Here's how the part is built. I have some questions about the finished solid (model axes, mm). A direction names the side the tool comes from. Coordinates: 2 decimals unless noted, no trailing zeros. Write each loop counter-clockwise with the first axis right and the second up, starting at its lowest first coordinate (ties: lowest second). Pieces come first, ordered by that corner, then holes. Notation, with made-up numbers: (69, 34.25) -> (116, 34.25) arc R23 cw to (116, 47.25) -> close; hole circle Ø7 at (11, -10). An arc over 180 degrees is marked (long way). Use a Markdown table: item, result. Add a question column.
Item 1: Will these pins go through, and if not, where does the flat tip stop? pin 1 Ø4 at (x, z) = (80.5, -6.5) entering from +Y; pin 2 Ø1.3 at (x, y) = (141.5, 9) entering from -Z; pin 3 Ø5 at (x, y) = (19, 14) entering from +Z.
Item 2: If I drill on line 1 along X through (y, z) = (0.35, 0); line 2 along Z through (x, y) = (35, 10.5); line 3 along Z through (x, y) = (78.5, 7.5), over which ranges is the centre line in solid material (lowest first)? Write a range as from..to.
Item 3: Imagine slicing it at B-B, the plane y = 16.5. Write out the boundary of the cut face in (x, z) (1 decimal).
Item 4: Imagine slicing it at A-A, the plane x = 106. Write out the boundary of the cut face in (y, z) (1 decimal), and give its area (3 significant figures).
Item 5: On a 3-axis mill with a long thin cutter (end or side, diameter ignored), from which of +Z, -Z, +X, -X, +Y, -Y can I reach the whole of each face in a straight line? I mean faces 5 (the flat face through (70, 10, -6.528)), 6 (the cylindrical face through (-10.38, 5.66, 7.59)), 7 (the cylindrical face through (133.184, 12.93, 7.146)). Say none if no direction works.
Item 6: If we mould it in two halves opening along Y, with no side actions, what happens to faces 1 (the flat face through (138, 18.136, 7)), 2 (the flat face through (140.64, 9, -3)), 3 (the flat face through (39, 7, -6.972)), 4 (the flat face through (38, 7, 6.972))? For each: pulls with the +Y half, pulls with the -Y half, needs draft (parallel to the pull), parting line crosses it, or undercut.
```python
from build123d import *

# Parameters (mm, degrees)
BOSS_EXTRUDE1_DEPTH          = 7.747
BOSS_EXTRUDE2_DEPTH          = 8.1915
SHELL1_START                 = 1.2192
SHELL1_DEPTH                 = 16.9164
CUT_EXTRUDE1_DEPTH           = 1.2192
EXTRUDE_THIN1_START          = -16.383
SKETCH4_W                    = 128.27
SKETCH4_H                    = 1.27
EXTRUDE_THIN1_DEPTH          = 16.383
FILLET1_R                    = 2.54
SKETCH5_W                    = 13.9446
SKETCH5_H                    = 1.27
CUT_EXTRUDE2_DEPTH           = 129.4892
F_3_4_0_162_DIAMETER_HOLE1_D = 4.1148
CUT_EXTRUDE3_REACH           = 145.248
FILLET2_DEPTH                = 18.1356
CUT_EXTRUDE4_REACH           = 145.099
SKETCH9_R                    = 2.9591
FILLET3_R                    = 0.635
FILLET4_R                    = 2.54


with BuildPart() as part:
    # Sketch1 → Boss-Extrude1 (new, symmetric)
    with BuildSketch(Plane.XY):
        with BuildLine():
            Line((0, 0), (141.859, 0))
            Line((141.859, 0), (141.859, 18.1356))
            Line((141.859, 18.1356), (133.9088, 18.1356))
            Line((133.9088, 18.1356), (133.9088, 12.1666))
            Line((133.9088, 12.1666), (129.615181762, 12.1666))
            ThreePointArc((129.615181762, 12.1666), (128.080397702, 13.170161892), (128.3843, 14.978570578))
            ThreePointArc((128.3843, 14.978570578), (128.72346749, 16.699838275), (127.341060995, 17.78))
            Line((127.341060995, 17.78), (124.186037439, 18.1356))
            Line((124.186037439, 18.1356), (121.646037439, 18.1356))
            Line((121.646037439, 18.1356), (108.629212725, 15.24))
            Line((108.629212725, 15.24), (8.934212725, 15.24))
            Line((8.934212725, 15.24), (0, 12.7))
            Line((0, 12.7), (0, 0))
        make_face()
    extrude(amount=BOSS_EXTRUDE1_DEPTH, both=True)

    # Sketch2 → Boss-Extrude2 (add, symmetric)
    with BuildSketch(Plane.XY):
        with BuildLine():
            Line((0, 12.7), (-7.024172619, 10.703025112))
            ThreePointArc((-7.024172619, 10.703025112), (-10.369324418, 5.571014033), (-5.748264059, 1.5494))
            Line((-5.748264059, 1.5494), (0, 1.5494))
            Line((0, 1.5494), (0, 12.7))
        make_face()
    extrude(amount=BOSS_EXTRUDE2_DEPTH, both=True)

    # Shell1: read off the stored shape, not the designer's step
    # Shell1 outline → Shell1 (cut)
    with BuildSketch(Plane(origin=(0, 0, 0), x_dir=(1, 0, 0), z_dir=(0, 1, 0)).offset(SHELL1_START)):
        Polygon((140.6398, -6.5278), (140.6398, 6.5278), (-1.2192, 6.5278), (-1.2192, 6.9723), (-12, 6.9723), (-12, -6.9723), (-1.2192, -6.9723), (-1.2192, -6.5278), align=None)
    extrude(amount=SHELL1_DEPTH, mode=Mode.SUBTRACT)

    # Sketch3 → Cut-Extrude1 (cut)
    with BuildSketch(Plane(origin=(141.859, 0, 0), x_dir=(0, 0, -1), z_dir=(1, 0, 0))):
        Polygon((-2.2225, 13.0556), (-0.635, 13.0556), (-0.635, 0), (0.635, 0), (0.635, 13.0556), (2.2225, 13.0556), (2.2225, 18.1356), (-2.2225, 18.1356), align=None)
    extrude(amount=-CUT_EXTRUDE1_DEPTH, mode=Mode.SUBTRACT)

    # Sketch4 → Extrude-Thin1 (add)
    with BuildSketch(Plane.XY.offset(8.1915).offset(EXTRUDE_THIN1_START)):
        with Locations((64.135, 7.1628)):
            Rectangle(SKETCH4_W, SKETCH4_H)
    extrude_thin1 = extrude(amount=EXTRUDE_THIN1_DEPTH)

    # Fillet1
    fillet1_edges = [part.edges().sort_by_distance(p)[0] for p in [
        (141.859, 9.0678, 7.747),
        (141.859, 9.0678, -7.747),
    ]]
    fillet(fillet1_edges, radius=FILLET1_R)

    # Mirror2: Extrude-Thin1 across plane
    add(extrude_thin1.mirror(Plane.XY))

    # Sketch5 → Cut-Extrude2 (cut)
    with BuildSketch(Plane.ZY.offset(1.2192)):
        with Locations((0, 7.1628)):
            Rectangle(SKETCH5_W, SKETCH5_H)
    extrude(amount=-CUT_EXTRUDE2_DEPTH, mode=Mode.SUBTRACT)

    # 3/4 (0.162) Diameter Hole1 (through all)
    with Locations(Plane(origin=(0, 0, -8.1915), x_dir=(-1, 0, 0), z_dir=(0, 0, -1))):
        with Locations((5.748264059, 6.215135941)):
            Hole(F_3_4_0_162_DIAMETER_HOLE1_D / 2)

    # Sketch8 → Cut-Extrude3 (cut, up to next)
    with BuildSketch(Plane.XZ, mode=Mode.PRIVATE) as cut_extrude3_sk1:
        Polygon((140.6398, -6.5278), (140.6398, 6.5278), (140.0048, 6.5278), (140.0048, 4.064), (133.9088, 4.064), (133.9088, -4.064), (140.0048, -4.064), (140.0048, -6.5278), align=None)
    cut_extrude3_tool1 = extrude(cut_extrude3_sk1.sketch, amount=-CUT_EXTRUDE3_REACH, mode=Mode.PRIVATE) & part.part
    add(cut_extrude3_tool1.solids().sort_by_distance((137.439195, 0, 0))[0], mode=Mode.SUBTRACT)

    # Fillet2: read off the stored shape, not the designer's step
    # Fillet2 outline → Fillet2 (add)
    with BuildSketch(Plane(origin=(0, 0, 0), x_dir=(1, 0, 0), z_dir=(0, 1, 0))):
        with BuildLine():
            ThreePointArc((140.0048, 6.5278), (140.453812806, 6.341812806), (140.6398, 5.8928))
            Line((140.6398, 5.8928), (140.6398, 6.5278))
            Line((140.6398, 6.5278), (140.0048, 6.5278))
        make_face()
        with BuildLine():
            Line((140.6398, -6.5278), (140.6398, -5.8928))
            ThreePointArc((140.6398, -5.8928), (140.453812806, -6.341812806), (140.0048, -6.5278))
            Line((140.0048, -6.5278), (140.6398, -6.5278))
        make_face()
    extrude(amount=FILLET2_DEPTH)

    # Sketch9 → Cut-Extrude4 (cut, up to next)
    with BuildSketch(Plane(origin=(0, 1.2192, 0), x_dir=(1, 0, 0), z_dir=(0, 1, 0)), mode=Mode.PRIVATE) as cut_extrude4_sk1:
        with Locations(Location((119.9388, 0, 0), (0, 0, 270))):
            Circle(SKETCH9_R)
    cut_extrude4_tool1 = extrude(cut_extrude4_sk1.sketch, amount=-CUT_EXTRUDE4_REACH, mode=Mode.PRIVATE) & part.part
    # Sketch9 → Cut-Extrude4 (cut, up to next)
    with BuildSketch(Plane(origin=(0, 1.2192, 0), x_dir=(1, 0, 0), z_dir=(0, 1, 0)), mode=Mode.PRIVATE) as cut_extrude4_sk2:
        with Locations(Location((6.985, 0, 0), (0, 0, 270))):
            Circle(SKETCH9_R)
    cut_extrude4_tool2 = extrude(cut_extrude4_sk2.sketch, amount=-CUT_EXTRUDE4_REACH, mode=Mode.PRIVATE) & part.part
    add(cut_extrude4_tool1.solids().sort_by_distance((119.9388, 1.2192, 0))[0], mode=Mode.SUBTRACT)
    add(cut_extrude4_tool2.solids().sort_by_distance((6.985, 1.2192, 0))[0], mode=Mode.SUBTRACT)

    # Fillet3
    fillet3_edges = [part.edges().sort_by_distance(p)[0] for p in [
        (141.859, 0, -2.921),
        (69.6595, 0, -7.747),
        (141.859, 0, 2.921),
        (141.115051224, 0, 7.003051224),
        (141.115051224, 0, -7.003051224),
        (69.6595, 0, 7.747),
    ]]
    fillet(fillet3_edges, radius=FILLET3_R)

    # Fillet4
    fillet4_edges = [part.edges().sort_by_distance(p)[0] for p in [
        (133.9088, 12.1666, 7.1374),
        (133.9088, 12.1666, -7.1374),
    ]]
    fillet(fillet4_edges, radius=FILLET4_R)


solid = part.part
```
Ans:
| question | item | result |
|---|---|---|
| 1 | pin 1 | stops at y = 15.24 |
| 1 | pin 2 | stops at z = -7.23 |
| 1 | pin 3 | stops at z = 7.75 |
| 2 | line 1 | x = 0..4.03, 9.94..116.98, 122.9..133.91 |
| 2 | line 2 | z = -7.75..-6.53, 6.53..7.75 |
| 2 | line 3 | z = -8.19..-6.97, 6.97..8.19 |
| 3 | outline | (114.3, -7.7) -> (128.8, -7.7) -> (128.8, -6.5) -> (114.3, -6.5) -> close; (114.3, 6.5) -> (128.8, 6.5) -> (128.8, 7.7) -> (114.3, 7.7) -> close; (133.9, -7.7) -> (139.3, -7.7) arc R2.5 ccw to (141.9, -5.2) -> (141.9, -2.2) -> (140.6, -2.2) -> (140.6, -5.9) arc R0.6 cw to (140, -6.5) -> (133.9, -6.5) -> close; (133.9, 6.5) -> (140, 6.5) arc R0.6 cw to (140.6, 5.9) -> (140.6, 2.2) -> (141.9, 2.2) -> (141.9, 5.2) arc R2.5 ccw to (139.3, 7.7) -> (133.9, 7.7) -> close |
| 4 | outline | (0, -7.1) arc R0.6 ccw to (0.6, -7.7) -> (6.5, -7.7) -> (6.5, -8.2) -> (7.8, -8.2) -> (7.8, -7.7) -> (15.2, -7.7) -> (15.2, -6.5) -> (7.8, -6.5) -> (7.8, -7) -> (6.5, -7) -> (6.5, -6.5) -> (1.2, -6.5) -> (1.2, 6.5) -> (6.5, 6.5) -> (6.5, 7) -> (7.8, 7) -> (7.8, 6.5) -> (15.2, 6.5) -> (15.2, 7.7) -> (7.8, 7.7) -> (7.8, 8.2) -> (6.5, 8.2) -> (6.5, 7.7) -> (0.6, 7.7) arc R0.6 ccw to (0, 7.1) -> close |
| 4 | area | 52.9 mm^2 |
| 5 | face 5 | -X, +Y |
| 5 | face 6 | +Z, -Z, -X |
| 5 | face 7 | +Z, -Z, +Y |
| 6 | face 1 | pulls with the +Y half |
| 6 | face 2 | needs draft |
| 6 | face 3 | undercut |
| 6 | face 4 | undercut |
